```python
from build123d import *

# Parameters (mm, degrees)
F0_R      = 26.35
F0_R_2    = 22.5
F1_DEPTH  = 25
F2_R      = 38.35
F2_R_2    = 26.35
F2_R_3    = 22.5
F3_DEPTH  = 2
F4_R      = 11
F5_DEPTH  = 25
F6_R      = 17.3263528998
F7_DEPTH  = 5
F8_R      = 11
F9_DEPTH  = 25
F10_W     = 19.7272742478
F10_H     = 3
F10_W_2   = 21.5454568693
F11_DEPTH = 1


with BuildPart() as f1:
    # F0 (on Top) → F1 (new body)
    with BuildSketch(Plane.XY):
        Circle(F0_R)
        Circle(F0_R_2, mode=Mode.SUBTRACT)
    extrude(amount=F1_DEPTH)

    # F2 (on face) → F3 (join)
    with BuildSketch(Plane(origin=(0, 0, 0), x_dir=(1, 0, 0), z_dir=(0, 0, -1))):
        Circle(F2_R)
        Circle(F2_R_2, mode=Mode.SUBTRACT)
        Circle(F2_R_2)
        Circle(F2_R_3, mode=Mode.SUBTRACT)
        Circle(F2_R_3)
    extrude(amount=F3_DEPTH)

    # F4 (on face) → F5 (cut)
    with BuildSketch(Plane(origin=(0, 0, -2), x_dir=(1, 0, 0), z_dir=(0, 0, -1))):
        Circle(F4_R)
    extrude(amount=-F5_DEPTH, mode=Mode.SUBTRACT)

    # F6 (on face) → F7 (join)
    with BuildSketch(Plane.XY):
        Circle(F6_R)
    extrude(amount=F7_DEPTH)

    # F8 (on face) → F9 (cut)
    with BuildSketch(Plane(origin=(0, 0, 0), x_dir=(1, 0, 0), z_dir=(0, 0, -1))):
        Circle(F8_R)
    extrude(amount=-F9_DEPTH, mode=Mode.SUBTRACT)

    # F10 (on face) → F11 (join)
    with BuildSketch(Plane.XY.offset(5)):
        with Locations((0.8293200467, 10)):
            Rectangle(F10_W, F10_H)
        with Locations((0.4202285782, -10)):
            Rectangle(F10_W_2, F10_H)
    extrude(amount=-F11_DEPTH)


solid = f1.part
```
Check sheet for the modelled part. Datum: model origin and axes. Units: mm. A direction names the side the tool comes from. Give positions to 0.01 mm unless a question says otherwise; leave off trailing zeros. Loops run counter-clockwise (first coordinate to the right, second up) from the corner with the lowest first, then second, coordinate; pieces in that order, holes last. Notation, with made-up numbers: M -19.5,-3.75 L -4.5,-3.75 A21 cw -4.5,24.25 Z; hole C -10,-39.5 d10. An arc over 180 degrees is marked long. Answer as CSV lines item,"result".
Item 1: Depth check by flat-ended pin: pin 1 Ø4 at (y, z) = (-4, 18) entering from +X; pin 2 Ø0.5 at (x, z) = (2, 4.5) entering from +Y; pin 3 Ø3 at (x, z) = (-13, 18.5) entering from -Y; pin 4 Ø3 at (x, y) = (3, -10.5) entering from -Z. Enter the tip coordinate at first touch or a pass-through.
Reply:
pin 1,"x = 26.27"
pin 2,"y = 26.29"
pin 3,"y = -23.71"
pin 4,"z = -2"
Item 2: Sectioned sample at C-C, the plane z = 13.5. Enter the section's corners in (x, y), then the cut area to 3 significant figures.
Reply:
outline,"C 0,0 d52.7; hole C 0,0 d45"
area,"591 mm^2"
Item 3: Scan lines: L1, parallel to Y at x = 0, z = 2.75; L2, parallel to Y at x = 0, z = 19; L3, parallel to X at y = -0.5, z = 9. Record each from-to range of solid material in increasing order.
Reply:
L1,"-26.35 to -22.5, -17.33 to -11, 11 to 17.33, 22.5 to 26.35"
L2,"-26.35 to -22.5, 22.5 to 26.35"
L3,"-26.35 to -22.49, 22.49 to 26.35"
Item 4: Sectioned sample at B-B, the plane x = 0. Enter the section's corners in (y, z).
Reply:
outline,"M -38.35,-2 L -11,-2 L -11,4 L -8.5,4 L -8.5,5 L -17.33,5 L -17.33,0 L -22.5,0 L -22.5,25 L -26.35,25 L -26.35,0 L -38.35,0 Z; M 8.5,4 L 11,4 L 11,-2 L 38.35,-2 L 38.35,0 L 26.35,0 L 26.35,25 L 22.5,25 L 22.5,0 L 17.33,0 L 17.33,5 L 8.5,5 Z"
Item 5: Set-up check for faces 1 (the face through (-11, 0, 1)), 2 (the face through (8, 8, -2)), 3 (the face through (-3.756, -16.914, 2.465)): record each of +Z, -Z, +X, -X, +Y, -Y from which the full face is reachable in a straight line by a thin tool's end or side.
Reply:
face 1,"-Z"
face 2,"-Z, +X, -X, +Y, -Y"
face 3,"+Z"
Item 6: Sectioned sample at A-A, the plane y = 0. Enter the section's corners in (x, z), then the cut area to 3 significant figures.
Reply:
outline,"M -38.35,-2 L -11,-2 L -11,5 L -17.33,5 L -17.33,0 L -22.5,0 L -22.5,25 L -26.35,25 L -26.35,0 L -38.35,0 Z; M 11,-2 L 38.35,-2 L 38.35,0 L 26.35,0 L 26.35,25 L 22.5,25 L 22.5,0 L 17.33,0 L 17.33,5 L 11,5 Z"
area,"365 mm^2"
Item 7: Sectioned sample at D-D, the plane x = -16. Enter the section's corners in (y, z), then the cut area to 3 significant figures.
Reply:
outline,"M -34.85,-2 L 34.85,-2 L 34.85,0 L 20.94,0 L 20.94,25 L 15.82,25 L 15.82,0 L 6.65,0 L 6.65,5 L -6.65,5 L -6.65,0 L -15.82,0 L -15.82,25 L -20.94,25 L -20.94,0 L -34.85,0 Z"
area,"462 mm^2"
